from build123d import *

# Parameters (mm, degrees)
SKETCH1_W           = 25
SKETCH1_H           = 52
BOSS_EXTRUDE1_DEPTH = 750
CUT_EXTRUDE2_DEPTH  = 40


with BuildPart() as part:
    # Sketch1 → Boss-Extrude1 (new body)
    with BuildSketch(Plane(origin=(0, 0, 0), x_dir=(1, 0, 0), z_dir=(0, 1, 0))):
        with Locations((-88.737623762, -4.094059406)):
            Rectangle(SKETCH1_W, SKETCH1_H)
    extrude(amount=BOSS_EXTRUDE1_DEPTH)

    # Sketch3 → Cut-Extrude2 (cut)
    with BuildSketch(Plane.ZY.offset(101.237623762)):
        with BuildLine():
            ThreePointArc((4.094059406, 58), (0.5585255, 56.535533906), (-0.905940594, 53))
            ThreePointArc((-0.905940594, 53), (0.5585255, 49.464466094), (4.094059406, 48))
            Line((4.094059406, 48), (4.094059406, 53))
            Line((4.094059406, 53), (4.094059406, 58))
        make_face()
        with BuildLine():
            ThreePointArc((9.094059406, 53), (7.629593312, 56.535533906), (4.094059406, 58))
            Line((4.094059406, 58), (4.094059406, 53))
            Line((4.094059406, 53), (4.094059406, 48))
            ThreePointArc((4.094059406, 48), (7.629593312, 49.464466094), (9.094059406, 53))
        make_face()
        with BuildLine():
            ThreePointArc((4.094059406, 58), (0.5585255, 56.535533906), (-0.905940594, 53))
            ThreePointArc((-0.905940594, 53), (0.5585255, 49.464466094), (4.094059406, 48))
            Line((4.094059406, 48), (4.094059406, 53))
            Line((4.094059406, 53), (4.094059406, 58))
        make_face()
        with BuildLine():
            ThreePointArc((9.094059406, 53), (7.629593312, 56.535533906), (4.094059406, 58))
            Line((4.094059406, 58), (4.094059406, 53))
            Line((4.094059406, 53), (4.094059406, 48))
            ThreePointArc((4.094059406, 48), (7.629593312, 49.464466094), (9.094059406, 53))
        make_face()
        with BuildLine():
            ThreePointArc((9.094059406, 394), (7.629593312, 390.464466094), (4.094059406, 389))
            Line((4.094059406, 389), (4.094059406, 58))
            ThreePointArc((4.094059406, 58), (7.629593312, 56.535533906), (9.094059406, 53))
            Line((9.094059406, 53), (9.094059406, 394))
        make_face()
        with BuildLine():
            ThreePointArc((4.094059406, 389), (0.5585255, 390.464466094), (-0.905940594, 394))
            Line((-0.905940594, 394), (-0.905940594, 53))
            ThreePointArc((-0.905940594, 53), (0.5585255, 56.535533906), (4.094059406, 58))
            Line((4.094059406, 58), (4.094059406, 389))
        make_face()
        with BuildLine():
            ThreePointArc((4.094059406, 399), (0.5585255, 397.535533906), (-0.905940594, 394))
            ThreePointArc((-0.905940594, 394), (0.5585255, 390.464466094), (4.094059406, 389))
            Line((4.094059406, 389), (4.094059406, 394))
            Line((4.094059406, 394), (4.094059406, 399))
        make_face()
        with BuildLine():
            ThreePointArc((9.094059406, 394), (7.629593312, 397.535533906), (4.094059406, 399))
            Line((4.094059406, 399), (4.094059406, 394))
            Line((4.094059406, 394), (4.094059406, 389))
            ThreePointArc((4.094059406, 389), (7.629593312, 390.464466094), (9.094059406, 394))
        make_face()
        with BuildLine():
            ThreePointArc((4.094059406, 399), (0.5585255, 397.535533906), (-0.905940594, 394))
            ThreePointArc((-0.905940594, 394), (0.5585255, 390.464466094), (4.094059406, 389))
            Line((4.094059406, 389), (4.094059406, 394))
            Line((4.094059406, 394), (4.094059406, 399))
        make_face()
        with BuildLine():
            ThreePointArc((9.094059406, 394), (7.629593312, 397.535533906), (4.094059406, 399))
            Line((4.094059406, 399), (4.094059406, 394))
            Line((4.094059406, 394), (4.094059406, 389))
            ThreePointArc((4.094059406, 389), (7.629593312, 390.464466094), (9.094059406, 394))
        make_face()
    extrude(amount=-CUT_EXTRUDE2_DEPTH, mode=Mode.SUBTRACT)


solid = part.part
Can you work these out from the model? Positions are in its coordinate system, mm. A direction names the side the tool comes from. Give positions to 0.01 mm unless a question says otherwise; leave off trailing zeros. Loops run counter-clockwise (first coordinate to the right, second up) from the corner with the lowest first, then second, coordinate; pieces in that order, holes last. Notation, with made-up numbers: M 22,55 L 80,55 A13 ccw 80,75 Z; hole C 82,-9 d6. An arc over 180 degrees is marked long. One line per item, written item: value. Start each with the question number.
1) If we section it at B-B, the plane y = 281: Write out the boundary of the cut face in (x, z).
2) If we section it at A-A, the plane x = -89: Write out the boundary of the cut face in (y, z).
3) I'm going to push a flat-ended pin straight in: pin 1 (1.5 mm diameter, centred on x = -81, z = 22.5, fed in from -Y). Where does the tip first touch, or does it pass through?
4) On a 3-axis mill with a long thin cutter (end or side, diameter ignored), from which of +Z, -Z, +X, -X, +Y, -Y can I reach the whole of each face in a straight line? I mean faces 1 (the face through (-101.238, 369.8, -1.3)), 2 (the face through (-89, 221, 9.094)). Say none if no direction works.
5) If I drill on line 1 (Z direction, x = -88.5, y = 337), over which ranges is the centre line in solid material (lowest first)? Write a range as [from, to].
6) Thinking about a two-plate mould opening in Y: for faces 3 (the face through (-89, 370, -21.906)), 4 (the face through (-89, 750, 4)), 5 (the face through (-89, 0, 4)), 6 (the face through (-89, 226, -0.906)), which applies, +Y half, -Y half, draft (parallel to the pull), parting line (faces both ways), or undercut?
Completed:
1. outline: M -101.24,-21.91 L -76.24,-21.91 L -76.24,-0.91 L -101.24,-0.91 Z; M -101.24,9.09 L -76.24,9.09 L -76.24,30.09 L -101.24,30.09 Z
2. outline: M 0,-21.91 L 750,-21.91 L 750,30.09 L 0,30.09 Z; hole M 53,-0.91 L 394,-0.91 A5 ccw 394,9.09 L 53,9.09 A5 ccw Z
3. pin 1: stops at y = 0
4. face 1: +Z, -Z, -X, +Y, -Y
4. face 2: +X, -X
5. line 1: z = [-21.91, -0.91], [9.09, 30.09]
6. face 3: draft
6. face 4: +Y half
6. face 5: -Y half
6. face 6: undercut
